```python
from build123d import *

# Parameters (mm, degrees)
F0_W      = 550
F0_H      = 63
F1_DEPTH  = 38
F2_W      = 38
F2_H      = 63
F3_DEPTH  = 2149
F4_W      = 38
F4_H      = 63
F5_DEPTH  = 2149
F6_W      = 38
F6_H      = 63
F7_DEPTH  = 2149
F8_W      = 1263.5
F8_H      = 63
F9_DEPTH  = 38
F10_W     = 63
F10_H     = 38
F11_DEPTH = 713.5
F12_W     = 38
F12_H     = 63
F13_DEPTH = 169


with BuildPart() as f1:
    # F0 (on Top) → F1 (new body)
    with BuildSketch(Plane.XY):
        with Locations((-275, 31.5)):
            Rectangle(F0_W, F0_H)
    extrude(amount=F1_DEPTH)

    # F2 (on face) → F3 (join)
    with BuildSketch(Plane.XY.offset(38)):
        with Locations((-531, 31.5)):
            Rectangle(F2_W, F2_H)
    extrude(amount=F3_DEPTH)

    # F4 (on face) → F5 (join)
    with BuildSketch(Plane.XY.offset(38)):
        with Locations((-19, 31.5)):
            Rectangle(F4_W, F4_H)
    extrude(amount=F5_DEPTH)

    # F6 (on face) → F7 (join)
    with BuildSketch(Plane.XY.offset(38)):
        with Locations((-275, 31.5)):
            Rectangle(F6_W, F6_H)
    extrude(amount=F7_DEPTH)

    # F8 (on face) → F9 (join)
    with BuildSketch(Plane.XY.offset(2187)):
        with Locations((-631.75, 31.5)):
            Rectangle(F8_W, F8_H)
    extrude(amount=F9_DEPTH)

    # F10 (on face) → F11 (join)
    with BuildSketch(Plane(origin=(-550, 0, 0), x_dir=(0, -1, 0), z_dir=(-1, 0, 0))):
        with Locations((-31.5, 1999)):
            Rectangle(F10_W, F10_H)
    extrude(amount=F11_DEPTH)

    # F12 (on face) → F13 (join)
    with BuildSketch(Plane.XY.offset(2018)):
        with Locations((-1244.5, 31.5)):
            Rectangle(F12_W, F12_H)
    extrude(amount=F13_DEPTH)


solid = f1.part
```
Design review of the part built by this model. Coordinates are the model's own, in mm. A direction names the side the tool comes from. Coordinates: 2 decimals unless noted, no trailing zeros. Write each loop counter-clockwise with the first axis right and the second up, starting at its lowest first coordinate (ties: lowest second). Pieces come first, ordered by that corner, then holes. Notation, with made-up numbers: M -13,-31 L -3,-31 A15 cw -3,-3 Z; hole C -25,45 d6. An arc over 180 degrees is marked long. Answer as a JSON object with one key per item and string values.
Item 1: Insertion check: pin 1 Ø19 at (y, z) = (22.5, 704) entering from -X. The pin has a flat end and moves straight along its axis. Give the tip position at first contact, or say it passes through.
Outcome:
{"pin 1": "x = -550"}
Item 2: Add section A-A, the plane x = -199.5. Give the boundary of the cut face in (y, z), and give its area (3 significant figures).
Outcome:
{"outline": "M 0,0 L 63,0 L 63,38 L 0,38 Z; M 0,2187 L 63,2187 L 63,2225 L 0,2225 Z", "area": "4,790 mm²"}
Item 3: Machinability: for faces 1 (the flat face through (-256, 31, 1097)), 2 (the flat face through (-902, 32, 1980)), 3 (the flat face through (-260, 63, 1190)), which of the approach directions +Z, -Z, +X, -X, +Y, -Y give a long, thin tool a straight path to every point of the face, cutting with its end or side? Answer none if there is none.
Outcome:
{"face 1": "+Y, -Y", "face 2": "-Z, -X, +Y, -Y", "face 3": "+Z, -Z, +X, -X, +Y"}
Item 4: Add section C-C, the plane z = 757.5. Give the boundary of the cut face in (x, y).
Outcome:
{"outline": "M -550,0 L -512,0 L -512,63 L -550,63 Z; M -294,0 L -256,0 L -256,63 L -294,63 Z; M -38,0 L 0,0 L 0,63 L -38,63 Z"}
Item 5: Add section B-B, the plane y = 49. Give the boundary of the cut face in (x, z), and give its area (3 significant figures).
Outcome:
{"outline": "M -1263.5,1980 L -550,1980 L -550,0 L 0,0 L 0,2225 L -1263.5,2225 Z; hole M -1225.5,2018 L -550,2018 L -550,2187 L -1225.5,2187 Z; hole M -512,38 L -294,38 L -294,2187 L -512,2187 Z; hole M -256,38 L -38,38 L -38,2187 L -256,2187 Z", "area": "347,000 mm²"}
Item 6: Draft analysis for pull direction X (two halves, no side actions). For faces 4 (the flat face through (-279, 32, 0)), 5 (the flat face through (-892, 32, 2187)), 6 (the flat face through (-149, 32, 2187)), 7 (the flat face through (0, 31, 1097)), state which applies: pulls with the +X half, pulls with the -X half, needs draft (parallel to the pull), parting line crosses it, or undercut.
Outcome:
{"face 4": "needs draft", "face 5": "undercut", "face 6": "undercut", "face 7": "pulls with the +X half"}
Item 7: Wall thickness on probe 1 along X at (y, z) = (40, 1231.5); probe 2 along X at (y, z) = (39.5, 2073.5); probe 3 along X at (y, z) = (14, 1999.5): over which ranges is each line inside the solid? List them lowest first.
Outcome:
{"probe 1": "-550 to -512, -294 to -256, -38 to 0", "probe 2": "-1263.5 to -1225.5, -550 to -512, -294 to -256, -38 to 0", "probe 3": "-1263.5 to -512, -294 to -256, -38 to 0"}
